from build123d import *

# Parameters (mm, degrees)
F0_R          = 25.4
F1_DEPTH      = 6.35
F2_R          = 23.8125
F3_DEPTH      = 12.7
F4_R          = 25.4
F5_DEPTH      = 6.35
F6_R          = 6.35
F7_DEPTH      = 25.401
F9_D          = 3.175
F9_DEPTH      = 3.175
F9_TIP        = 0.9538662327
F10_S5_R      = 25.4
F10_T6_DEPTH  = 42
F10_S11_R     = 25.4
F10_T12_DEPTH = 40


# Not quite as in the source:
# - a fillet or chamfer that OpenCascade refuses, or shapes differently, is made with other operations: its cross-section is extruded or revolved along the edge and cut away or added


with BuildPart() as f1:
    # F0 (on Front) → F1 (new body)
    with BuildSketch(Plane.XZ):
        Circle(F0_R)
    extrude(amount=F1_DEPTH)

    # F2 (on face) → F3 (join)
    with BuildSketch(Plane.XZ.offset(6.35)):
        Circle(F2_R)
    extrude(amount=F3_DEPTH)

    # F4 (on face) → F5 (join)
    with BuildSketch(Plane.XZ.offset(19.05)):
        Circle(F4_R)
    extrude(amount=F5_DEPTH)

    # F6 (on face) → F7 (cut, through all)
    with BuildSketch(Plane.XZ.offset(25.4)):
        Circle(F6_R)
    extrude(amount=-F7_DEPTH, mode=Mode.SUBTRACT)

    # F9
    with Locations(Plane.XZ.offset(25.4)):
        with Locations((0, 19.05), (0, -19.05), (-19.05, 0), (19.05, 0)):
            Hole(F9_D / 2, depth=F9_DEPTH)
            with Locations((0, 0, -(F9_DEPTH + F9_TIP / 2))):  # 118° drill point
                Cone(0, F9_D / 2, F9_TIP, mode=Mode.SUBTRACT)

    # F10: fillet of radius 1.6002 on 5 edges, made by hand


with BuildPart() as f10_tool2:
    # F10_s3 → F10_t4 (revolve)
    with BuildSketch(Plane.XY):
        with BuildLine():
            ThreePointArc((23.8125, -7.9502), (24.2811877287, -6.8186877287), (25.4127, -6.35))
            Line((25.4127, -6.35), (23.8125, -6.35))
            Line((23.8125, -6.35), (23.8125, -7.9502))
        make_face()
    revolve(axis=Axis((0, -6.35, 0), (0, -1, 0)))

    # F10_s5 → F10_t6 (intersect, symmetric)
    with BuildSketch(Plane.XZ.offset(7.2)):
        Circle(F10_S5_R)
    extrude(amount=F10_T6_DEPTH, both=True, mode=Mode.INTERSECT)


with BuildPart() as f1_1:
    add(f1.part)

    # F10_t1: union F10_tool2
    add(f10_tool2.part)


with BuildPart() as f10_tool8:
    # F10_s9 → F10_t10 (revolve)
    with BuildSketch(Plane.XY):
        with BuildLine():
            ThreePointArc((25.4127, -19.05), (24.2811877287, -18.5813122713), (23.8125, -17.4498))
            Line((23.8125, -17.4498), (23.8125, -19.05))
            Line((23.8125, -19.05), (25.4127, -19.05))
        make_face()
    revolve(axis=Axis((0, -19.05, 0), (0, -1, 0)))

    # F10_s11 → F10_t12 (intersect, symmetric)
    with BuildSketch(Plane.XZ.offset(17.7)):
        Circle(F10_S11_R)
    extrude(amount=F10_T12_DEPTH, both=True, mode=Mode.INTERSECT)


with BuildPart() as f1_2:
    add(f1_1.part)

    # F10_t7: union F10_tool8
    add(f10_tool8.part)

    # F10_s13 → F10_t14 (revolve, cut)
    with BuildSketch(Plane.XY):
        with BuildLine():
            ThreePointArc((25.4, -23.7998), (24.9313122713, -24.9313122713), (23.7998, -25.4))
            Line((23.7998, -25.4), (25.4, -25.4))
            Line((25.4, -25.4), (25.4, -23.7998))
        make_face()
    revolve(axis=Axis((0, -25.4, 0), (0, -1, 0)), mode=Mode.SUBTRACT)

    # F10_s15 → F10_t16 (revolve, cut)
    with BuildSketch(Plane.XY):
        with BuildLine():
            ThreePointArc((23.7998, 0), (24.9313122713, -0.4686877287), (25.4, -1.6002))
            Line((25.4, -1.6002), (25.4, 0))
            Line((25.4, 0), (23.7998, 0))
        make_face()
    revolve(axis=Axis((0, 0, 0), (0, -1, 0)), mode=Mode.SUBTRACT)


solid = f1_2.part
Can you work these out from the model? Positions are in its coordinate system, mm. A direction names the side the tool comes from. Give positions to 0.01 mm unless a question says otherwise; leave off trailing zeros. Loops run counter-clockwise (first coordinate to the right, second up) from the corner with the lowest first, then second, coordinate; pieces in that order, holes last. Notation, with made-up numbers: (-9.75, 57) - (3.25, 57) arc R24 cw to (3.25, 85) - close; hole circle Ø3 at (18.5, 28.5). An arc over 180 degrees is marked (long way). Return JSON: item names as keys, results as strings.
1. I want a section at B-B on y = -2.5. Please give me the cut outline in (x, z), and give its area (3 significant figures).
Output values:
{"outline": "circle Ø50.8 at (0, 0); hole circle Ø12.7 at (0, 0)", "area": "1,900 mm²"}
2. For faces 4 (the face through (-5.506, -21.458, -24.796)), 5 (the face through (-18.897, -12.634, -14.49)), 6 (the face through (20.636, -23.79, 0.07)), which set-ups out of +Z, -Z, +X, -X, +Y, -Y let a thin tool reach every point of the face, with its end or its side?
Output values:
{"face 4": "+Y, -Y", "face 5": "none", "face 6": "-Y"}
3. If I drill on line 1 (Z direction, x = 0, y = -22.95); line 2 (Z direction, x = 0, y = -15); line 3 (Z direction, x = 5.5, y = -11.75), over which ranges is the centre line in solid material (lowest first)?
Output values:
{"line 1": "z = -25.4 to -20.64, -17.46 to -6.35, 6.35 to 17.46, 20.64 to 25.4", "line 2": "z = -23.81 to -6.35, 6.35 to 23.81", "line 3": "z = -23.17 to -3.17, 3.17 to 23.17"}
4. I'm going to push flat-ended pins straight in: pin 1 Ø1.9 at (x, z) = (-19.05, 0) entering from -Y; pin 2 Ø1.5 at (y, z) = (-8.5, 17.5) entering from -X; pin 3 Ø8 at (y, z) = (-18, 18) entering from -X; pin 4 Ø5 at (x, z) = (0, -19.05) entering from +Y. Where does each tip first touch, or does it pass through?
Output values:
{"pin 1": "stops at y = -21.84", "pin 2": "stops at x = -16.93", "pin 3": "stops at x = -21.1", "pin 4": "stops at y = 0"}
5. We'd pull the mould along X, two halves only. Please class faces 1 (the face through (-5.506, -4.008, -24.796)), 2 (the face through (0.34, -23.79, 17.5)), 3 (the face through (5, 0, -5)): +X half, -X half, draft (parallel to the pull), parting line (faces both ways), or undercut.
Output values:
{"face 1": "parting line", "face 2": "undercut", "face 3": "draft"}
